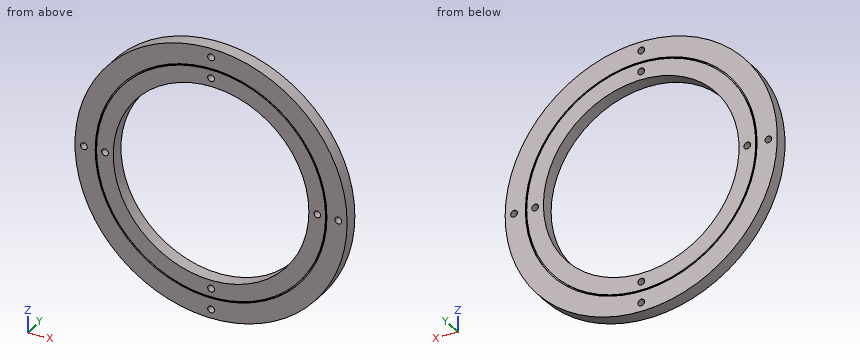
```python
from build123d import *

# Parameters (mm, degrees)
SKETCH1_R           = 101.0285
SKETCH1_R_2         = 72.6313
BOSS_EXTRUDE1_DEPTH = 10
SKETCH2_R           = 2.5
CUT_EXTRUDE1_DEPTH  = 11
SKETCH3_R           = 86.0285
SKETCH3_R_2         = 85.0285
CUT_EXTRUDE2_DEPTH  = 1


with BuildPart() as part:
    # Sketch1 → Boss-Extrude1 (new body)
    with BuildSketch(Plane(origin=(0, 0, 0), x_dir=(1, 0, 0), z_dir=(0, 1, 0))):
        Circle(SKETCH1_R)
        Circle(SKETCH1_R_2, mode=Mode.SUBTRACT)
    extrude(amount=BOSS_EXTRUDE1_DEPTH)

    # Sketch2 → Cut-Extrude1 (cut, through all)
    with BuildSketch(Plane(origin=(0, 10, 0), x_dir=(1, 0, 0), z_dir=(0, 1, 0))):
        with Locations((-94.4137, 0)):
            Circle(SKETCH2_R)
        with Locations((-78.7635, 0)):
            Circle(SKETCH2_R)
        with Locations((0, 78.7635)):
            Circle(SKETCH2_R)
        with Locations((0, 94.4137)):
            Circle(SKETCH2_R)
        with Locations((78.7635, 0)):
            Circle(SKETCH2_R)
        with Locations((94.4137, 0)):
            Circle(SKETCH2_R)
        with Locations((0, -78.7635)):
            Circle(SKETCH2_R)
        with Locations((0, -94.4137)):
            Circle(SKETCH2_R)
    extrude(amount=-CUT_EXTRUDE1_DEPTH, mode=Mode.SUBTRACT)

    # Sketch3 → Cut-Extrude2 (cut)
    with BuildSketch(Plane(origin=(0, 10, 0), x_dir=(1, 0, 0), z_dir=(0, 1, 0))):
        Circle(SKETCH3_R)
        Circle(SKETCH3_R_2, mode=Mode.SUBTRACT)
    cut_extrude2 = extrude(amount=-CUT_EXTRUDE2_DEPTH, mode=Mode.SUBTRACT)

    # Mirror1: Cut-Extrude2 across plane
    add(cut_extrude2.mirror(Plane.ZX.offset(5)), mode=Mode.SUBTRACT)


solid = part.part
```
Source: CAD feature listing. Evaluate the final solid. Frame: model axes, mm. Coordinates: 2 decimals unless noted, no trailing zeros. Loops run counter-clockwise (first coordinate to the right, second up) from the corner with the lowest first, then second, coordinate; pieces in that order, holes last. Notation, with made-up numbers: (35.5, -24) -> (77.5, -24) arc R19 cw to (77.5, -20) -> close; hole circle Ø3 at (44.25, 79.5). An arc over 180 degrees is marked (long way). One line per item, written item: value. Start each with the question number.
Q1. Section query B-B, the plane z = -29. Return the cut outline in (x, y), and give its area (3 significant figures).
Q2. Section query A-A, the plane x = 14.5. Return the cut outline in (y, z).
Q3. Section query C-C, the plane y = 3.5. Give the number of separate pieces and of enclosed holes in the cut face, and give its area (3 significant figures).
Q4. Line query: line 1 along X through (y, z) = (5, 0); line 2 along X through (y, z) = (9.5, -47). Output: solid intervals per line, ascending.
Q5. Contact query for flat-ended pins moving along their axis: P1, Ø5, axis at x = -37.5, y = 8.5, coming from the -Z side; P2, Ø4.5, axis at x = 78.76, z = 0, coming from the -Y side; P3, Ø2, axis at x = -60.5, y = 7.5, coming from the -Z side; P4, Ø1, axis at x = 6.5, y = 6, coming from the -Z side. Output: stop coordinate, or through.
Results:
1. outline: (-96.78, 0) -> (-80.99, 0) -> (-80.99, 1) -> (-79.93, 1) -> (-79.93, 0) -> (-66.59, 0) -> (-66.59, 10) -> (-79.93, 10) -> (-79.93, 9) -> (-80.99, 9) -> (-80.99, 10) -> (-96.78, 10) -> close; (66.59, 0) -> (79.93, 0) -> (79.93, 1) -> (80.99, 1) -> (80.99, 0) -> (96.78, 0) -> (96.78, 10) -> (80.99, 10) -> (80.99, 9) -> (79.93, 9) -> (79.93, 10) -> (66.59, 10) -> close
1. area: 599 mm^2
2. outline: (0, -99.98) -> (10, -99.98) -> (10, -84.8) -> (9, -84.8) -> (9, -83.78) -> (10, -83.78) -> (10, -71.17) -> (0, -71.17) -> (0, -83.78) -> (1, -83.78) -> (1, -84.8) -> (0, -84.8) -> close; (0, 71.17) -> (10, 71.17) -> (10, 83.78) -> (9, 83.78) -> (9, 84.8) -> (10, 84.8) -> (10, 99.98) -> (0, 99.98) -> (0, 84.8) -> (1, 84.8) -> (1, 83.78) -> (0, 83.78) -> close
3. separate pieces: 1
3. enclosed holes: 9
3. area: 15,300 mm^2
4. line 1: -101.03 to -96.91, -91.91 to -81.26, -76.26 to -72.63, 72.63 to 76.26, 81.26 to 91.91, 96.91 to 101.03
4. line 2: -89.43 to -72.05, -70.86 to -55.37, 55.37 to 70.86, 72.05 to 89.43
5. P1: z = -94.77
5. P2: through
5. P3: z = -81.65
5. P4: z = -100.85
